from build123d import *

# Parameters (mm, degrees)
CORTAR_EXTRUIR1_DEPTH = 10
CROQUIS3_R            = 11
CORTAR_EXTRUIR3_DEPTH = 9.5


# Read off the part's stored shape, not the designer's step: Vaciado4
with BuildPart() as part:
    # Croquis1 → Revolución1 (revolve)
    with BuildSketch(Plane.XY, mode=Mode.PRIVATE) as revoluci_n1_sk:
        with BuildLine():
            Line((-22.7696793, 0), (-22.7696793, 10))
            ThreePointArc((-22.7696793, 10), (-20.905680237, 11.112669164), (-18.7696793, 11.5))
            ThreePointArc((-18.7696793, 11.5), (-16.865736024, 11.109200978), (-15.2696793, 10))
            Line((-15.2696793, 10), (-11.2696793, 10))
            Line((-11.2696793, 10), (-11.2696793, 0))
            Line((-11.2696793, 0), (-22.7696793, 0))
        make_face()
    revolve(revoluci_n1_sk.sketch.rotate(Axis((-11.2696793, 0, 0), (0, 1, 0)), 270), axis=Axis((-11.2696793, 0, 0), (0, 1, 0)))

    # Croquis2 → Cortar-Extruir1 (cut)
    with BuildSketch(Plane(origin=(0, 10, 0), x_dir=(1, 0, 0), z_dir=(0, 1, 0))):
        with BuildLine():
            Line((-15.198737712, 0.75), (-7.340620889, 0.75))
            ThreePointArc((-7.340620889, 0.75), (-11.2696793, 4), (-15.198737712, 0.75))
        make_face()
        with BuildLine():
            Line((-15.198737712, -0.75), (-7.340620889, -0.75))
            ThreePointArc((-7.340620889, -0.75), (-11.2696793, -4), (-15.198737712, -0.75))
        make_face()
    extrude(amount=-CORTAR_EXTRUIR1_DEPTH, mode=Mode.SUBTRACT)

    # Croquis3 → Cortar-Extruir3 (cut)
    with BuildSketch(Plane.XZ):
        with Locations(Location((-11.2696793, 0, 0), (0, 0, 270))):
            Circle(CROQUIS3_R)
    extrude(amount=-CORTAR_EXTRUIR3_DEPTH, mode=Mode.SUBTRACT)

    # Vaciado4 outline → Vaciado4 (revolve, cut)
    with BuildSketch(Plane(origin=(-11.2696793, 0, 0), x_dir=(1, 0, 0), z_dir=(0, 0, 1))):
        with BuildLine():
            Line((10.5, 9.5), (10.5, 9.520357417))
            ThreePointArc((10.5, 9.520357417), (9.077949586, 10.248886951), (7.5, 10.5))
            ThreePointArc((7.5, 10.5), (6.166764081, 10.260679247), (5, 9.572599296))
            Line((5, 9.572599296), (5, 9.5))
            Line((5, 9.5), (10.5, 9.5))
        make_face()
    revolve(axis=Axis((-11.2696793, 0, 0), (0, 1, 0)), mode=Mode.SUBTRACT)


solid = part.part
Verification items for the finished model (mm, model axes). A direction names the side the tool comes from. Give positions to 0.01 mm unless a question says otherwise; leave off trailing zeros. Write each loop counter-clockwise with the first axis right and the second up, starting at its lowest first coordinate (ties: lowest second). Pieces come first, ordered by that corner, then holes. Notation, with made-up numbers: M 60,-8 L 71,-8 A23 cw 71,29 Z; hole C 6.25,28.25 d8. An arc over 180 degrees is marked long. Put each result on its own line as item: value. Start each with the question number.
1. Scan lines: line 1 along X through (y, z) = (5.25, 0); line 2 along X through (y, z) = (4, 10); line 3 along Z through (x, y) = (-7.75, 5). Record each from-to range of solid material in increasing order. Write a range as [from, to].
2. Draft check along Z on faces 3 (the face through (0, 0, 1)), 4 (the face through (-15, 9.5, -10)), 5 (the face through (-22.67, 5.07, 1.5)). Enter one of: +Z half, -Z half, draft (parallel to the pull), parting line (faces both ways), or undercut.
3. Go/stop test with flat-tipped pins: pin 1 Ø0.8 at (x, z) = (-13, 0) entering from +Y; pin 2 Ø6 at (x, z) = (-2, -5.5) entering from +Y; pin 3 Ø3 at (x, y) = (-17.5, 7) entering from +Z. Record where each tip stops, or that it passes through.
4. Section check B-B (x = -10.75). Give the number of separate pieces and of enclosed holes in the cut face, and give its area (3 significant figures).
5. Set-up check for faces 1 (the face through (-22.01, 4.68, 2.38)), 2 (the face through (-11, 10, 0)): record each of +Z, -Z, +X, -X, +Y, -Y from which the full face is reachable in a straight line by a thin tool's end or side.
6. Section check C-C (y = 1.5). Record the cut outline in (x, z), and give its area (3 significant figures).
Answer list:
1. line 1: [-22.77, -22.27], [-0.27, 0.23]
1. line 2: [-16.95, -15.85], [-6.69, -5.59]
1. line 3: [-10.95, -10.42], [10.42, 10.95]
2. face 3: draft
2. face 4: undercut
2. face 5: parting line
3. pin 1: y = 10
3. pin 2: y = 11.49
3. pin 3: z = 10.48
4. separate pieces: 3
4. enclosed holes: 0
4. area: 25.6 mm2
5. face 1: -Y
5. face 2: +Y
6. outline: C -11.27,0 d23; hole C -11.27,0 d22
6. area: 35.3 mm2
